```python
from build123d import *

# Parameters (mm, degrees)
F2_DEPTH = 9.144
F0_W     = 104.3482013047
F0_H     = 147.1950858831
F3_DEPTH = 1.016
F5_DEPTH = 8.128


with BuildPart() as f2:
    # F1 (on face) → F2 (new body)
    with BuildSketch(Plane.XY):
        Polygon((-44.0127886832, 33.2340672612), (-17.0306321234, 33.2340672612), (-17.0306321234, -24.6169902384), (-44.0127886832, -24.6169902384), (-44.0127886832, -73.8890171051), (60.3354126215, -73.8890171051), (60.3354126215, 73.306068778), (-44.0127886832, 73.306068778), align=None)
        Polygon((33.4283486009, -24.867111817), (33.4283486009, 33.2340672612), (59.7827173769, 33.2340672612), (60.2132864296, -24.867111817), align=None, mode=Mode.SUBTRACT)
    extrude(amount=F2_DEPTH)

    # F0 (on Top) + F2_face (on face) → F3 (join)
    with BuildSketch(Plane.XY):
        with Locations((8.1613119692, -0.2914741635)):
            Rectangle(F0_W, F0_H)
    with BuildSketch(Plane(origin=(8.2321469679, -1.4312137142, 9.144), x_dir=(1, 0, 0), z_dir=(0, 0, 1))):
        Polygon((-52.2449356511, 34.6652809755), (-25.2627790912, 34.6652809755), (-25.2627790912, -23.1857765242), (-52.2449356511, -23.1857765242), (-52.2449356511, -72.4578033909), (52.1032656536, -72.4578033909), (52.1032656536, 74.7372824923), (-52.2449356511, 74.7372824923), align=None)
        Polygon((51.9811394618, -23.4358981028), (25.196201633, -23.4358981028), (25.196201633, 34.6652809755), (51.5505704091, 34.6652809755), align=None, mode=Mode.SUBTRACT)
    extrude(amount=-F3_DEPTH)

    # F4 (on face) → F5 (join)
    with BuildSketch(Plane.XY.offset(9.144)):
        Polygon((59.7827173769, 33.2340672612), (33.4283486009, 33.2340672612), (33.4283486009, -24.867111817), (60.2132864296, -24.867111817), align=None)
    extrude(amount=-F5_DEPTH)


solid = f2.part
```
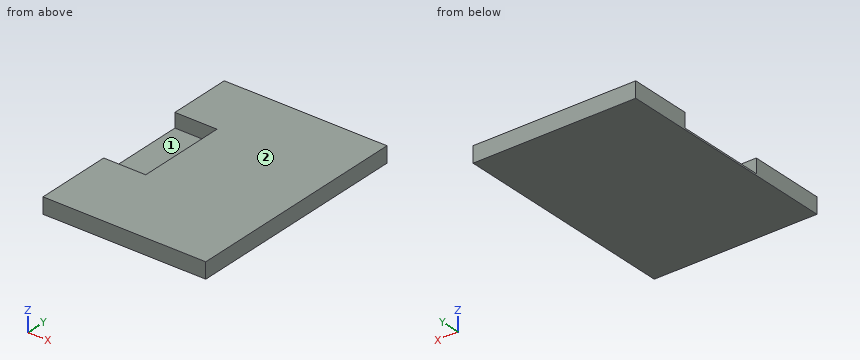
Verification items for the finished model (mm, model axes). Face numbers are marked on the shaded views. Give positions to 0.01 mm unless a question says otherwise; leave off trailing zeros. Loops run counter-clockwise (first coordinate to the right, second up) from the corner with the lowest first, then second, coordinate; pieces in that order, holes last.
1. Section check C-C, the plane z = 6.5. Enter the section's corners in (x, y).
2. Section check D-D, the plane y = -22. Enter the section's corners in (x, z), then the cut area to 3 significant figures.
3. Mould release check, pull along Y, two halves, no side actions. Record for the marked faces 1 and 2: released by +Y, released by -Y, zero draft, split by the parting line, or undercut.
4. Go/stop test with flat-tipped pins: pin 1 Ø2.5 at (y, z) = (2.5, 4.5) entering from -X; pin 2 Ø13.5 at (x, y) = (-36.5, -6) entering from +Z. Record where each tip stops, or that it passes through.
5. Section check B-B, the plane y = 4.5. Enter the section's corners in (x, z).
6. Thickness scan on line 1 (Z direction, x = 52, y = 20.5); line 2 (Y direction, x = -35.5, z = 3.75); line 3 (X direction, y = 23, z = 7). Record the ranges inside material, lowest first.
7. Section check A-A, the plane x = 54.5. Enter the section's corners in (y, z).
Geometry says:
1. outline: (-44.01, -73.89) - (60.34, -73.89) - (60.34, 73.31) - (-44.01, 73.31) - (-44.01, 33.23) - (-17.03, 33.23) - (-17.03, -24.62) - (-44.01, -24.62) - close
2. outline: (-44.01, -1.02) - (60.34, -1.02) - (60.34, 9.14) - (-17.03, 9.14) - (-17.03, 0) - (-44.01, 0) - close; hole (33.43, 0) - (60.19, 0) - (60.19, 1.02) - (33.43, 1.02) - close
2. area: 786 mm2
3. face 1: undercut
3. face 2: zero draft
4. pin 1: stops at x = -17.03
4. pin 2: stops at z = 0
5. outline: (-44.01, -1.02) - (60.34, -1.02) - (60.34, 9.14) - (-17.03, 9.14) - (-17.03, 0) - (-44.01, 0) - close; hole (33.43, 0) - (60, 0) - (60, 1.02) - (33.43, 1.02) - close
6. line 1: z = -1.02 to 0, 1.02 to 9.14
6. line 2: y = -73.89 to -24.62, 33.23 to 73.31
6. line 3: x = -17.03 to 60.34
7. outline: (-73.89, -1.02) - (73.31, -1.02) - (73.31, 9.14) - (-73.89, 9.14) - close; hole (-24.87, 0) - (33.23, 0) - (33.23, 1.02) - (-24.87, 1.02) - close
